Check sheet for the modelled part. Datum: model origin and axes. Units: mm. Coordinates: 2 decimals unless noted, no trailing zeros. Write each loop counter-clockwise with the first axis right and the second up, starting at its lowest first coordinate (ties: lowest second). Pieces come first, ordered by that corner, then holes. Notation, with made-up numbers: (27, -24.75) - (33, -24.75) arc R9 ccw to (33, -15.75) - close; hole circle Ø10 at (-2, -15.75). An arc over 180 degrees is marked (long way). Use one line per item in the form item = value. Start each with the question number.
1. Cross-section at A-A on x = 44.45. Record the boundary of the cut face in (y, z).
2. Go/stop test with flat-tipped pins: pin 1 Ø1.9 at (x, z) = (96, 2) entering from -Y; pin 2 Ø1.9 at (y, z) = (-4, 3.5) entering from -X. Record where each tip stops, or that it passes through.
3. Cross-section at B-B on z = 4. Give the number of separate pieces and of enclosed holes in the cut face, then the cut area to 3 significant figures.
4. Scan lines: line 1 along X through (y, z) = (40.88, 3.25); line 2 along X through (y, z) = (55.88, 3.5); line 3 along Y through (x, z) = (44.45, 1.75). Record each from-to range of solid material in increasing order.
```python
from build123d import *

# Parameters (mm, degrees)
SKETCH1_R           = 1.0922
SKETCH1_R_2         = 0.8
BOSS_EXTRUDE1_DEPTH = 6.35
FILLET1_R           = 10.16


with BuildPart() as part:
    # Sketch1 → Boss-Extrude1 (new body)
    with BuildSketch(Plane.XY):
        Polygon((88.9, 0), (101.6, 0), (101.6, 76.2), (0, 76.2), (0, 0), (12.7, 0), (12.7, -12.7), (88.9, -12.7), align=None)
        with Locations((44.45, 53.34)):
            Circle(SKETCH1_R, mode=Mode.SUBTRACT)
        with Locations(Location((57.15, 53.34, 0), (0, 0, 180))):
            Circle(SKETCH1_R, mode=Mode.SUBTRACT)
        with Locations((32.3, 55.88)):
            Circle(SKETCH1_R_2, mode=Mode.SUBTRACT)
        with Locations(Location((69.3, 55.88, 0), (0, 0, 180))):
            Circle(SKETCH1_R_2, mode=Mode.SUBTRACT)
        with Locations((32.125311619, 40.88)):
            Circle(SKETCH1_R_2, mode=Mode.SUBTRACT)
        with Locations(Location((69.474688381, 40.88, 0), (0, 0, 180))):
            Circle(SKETCH1_R_2, mode=Mode.SUBTRACT)
        with Locations((29.4386, 53.34)):
            Circle(SKETCH1_R_2, mode=Mode.SUBTRACT)
        with Locations((29.263911619, 35.9540048)):
            Circle(SKETCH1_R_2, mode=Mode.SUBTRACT)
        with Locations(Location((72.336088381, 35.9540048, 0), (0, 0, 180))):
            Circle(SKETCH1_R_2, mode=Mode.SUBTRACT)
        with Locations(Location((72.1614, 53.34, 0), (0, 0, 180))):
            Circle(SKETCH1_R_2, mode=Mode.SUBTRACT)
    extrude(amount=BOSS_EXTRUDE1_DEPTH)

    # Fillet1
    fillet1_edges = [part.edges().sort_by_distance(p)[0] for p in [
        (0, 76.2, 3.175),
        (101.6, 76.2, 3.175),
    ]]
    fillet(fillet1_edges, radius=FILLET1_R)


solid = part.part
```
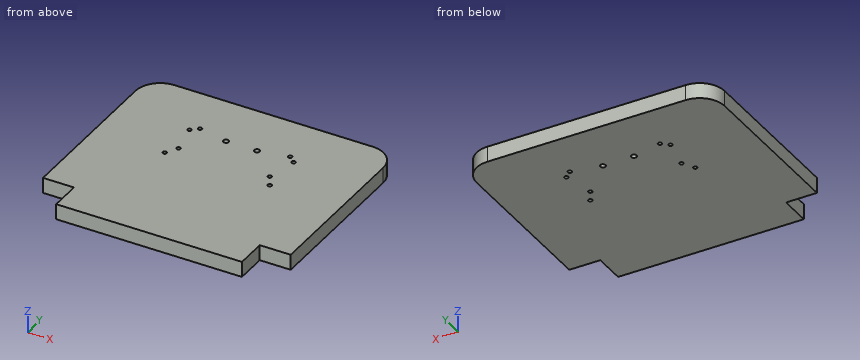
Final values:
q1.outline = (-12.7, 0) - (52.25, 0) - (52.25, 6.35) - (-12.7, 6.35) - close; (54.43, 0) - (76.2, 0) - (76.2, 6.35) - (54.43, 6.35) - close
q2.pin_1 = 0
q2.pin_2 = 12.7
q3.separate_pieces = 1
q3.enclosed_holes = 10
q3.area = 8,640 mm²
q4.line_1 = 0 to 31.33, 32.93 to 68.67, 70.27 to 101.6
q4.line_2 = 0 to 31.5, 33.1 to 68.5, 70.1 to 101.6
q4.line_3 = -12.7 to 52.25, 54.43 to 76.2
